Verification items for the finished model (mm, model axes). Face numbers are marked on the shaded views. Give positions to 0.01 mm unless a question says otherwise; leave off trailing zeros. Loops run counter-clockwise (first coordinate to the right, second up) from the corner with the lowest first, then second, coordinate; pieces in that order, holes last. Notation, with made-up numbers: (69, -40) - (103, -40) arc R22 cw to (103, -3) - close; hole circle Ø6 at (49.25, -5). An arc over 180 degrees is marked (long way). Put each result on its own line as item: value. Start each with the question number.
```python
from build123d import *

# Parameters (mm, degrees)
F0_W     = 50
F0_H     = 24
F0_R     = 2.75
F1_DEPTH = 4
F2_SIZE  = 7.62


with BuildPart() as f1:
    # F0 (on Top) → F1 (new body)
    with BuildSketch(Plane.XY):
        Rectangle(F0_W, F0_H)
        with Locations((-12.5, 0)):
            Circle(F0_R, mode=Mode.SUBTRACT)
        with BuildLine():
            ThreePointArc((15.2468, 0), (12.4968, -2.75), (9.7468, 0))
            ThreePointArc((9.7468, 0), (12.4968, 2.75), (15.2468, 0))
        make_face(mode=Mode.SUBTRACT)
    extrude(amount=F1_DEPTH)

    # F2
    f2_edges = [f1.edges().sort_by_distance(p)[0] for p in [
        (-25, 12, 2),
        (-25, -12, 2),
        (25, -12, 2),
        (25, 12, 2),
    ]]
    chamfer(f2_edges, length=F2_SIZE)


solid = f1.part
```
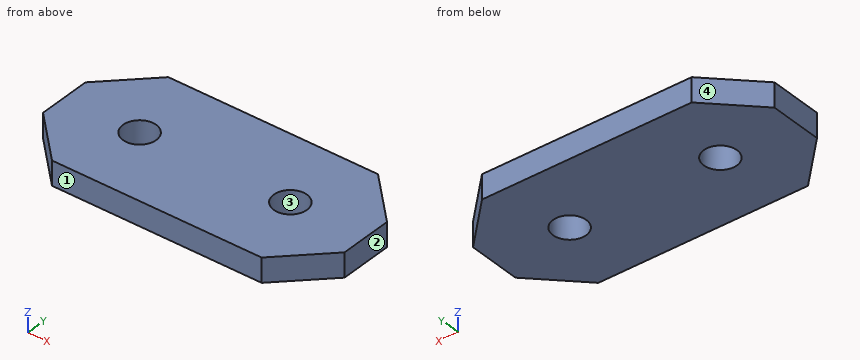
1) Section check B-B, the plane z = 2.7. Enter the section's corners in (x, y).
2) Depth check by flat-ended pin: P1, Ø7, axis at x = 12.5, y = 0, coming from the -Z side; P2, Ø4.5, axis at x = -12.5, y = 0, coming from the +Z side. Enter the tip coordinate at first touch or a pass-through.
3) Draft check along X on the marked faces 1, 2, 3 and 4. Enter one of: pulls with the +X half, pulls with the -X half, needs draft (parallel to the pull), parting line crosses it, or undercut.
4) Section check C-C, the plane x = -12.5. Enter the section's corners in (y, z).
5) Section check D-D, the plane y = 8.75. Enter the section's corners in (x, z).
6) Scan lines: line 1 along Y through (x, z) = (-12.5, 1.35); line 2 along X through (y, z) = (-0.75, 2.55); line 3 along Y through (x, z) = (-15, 1.8). Record each from-to range of solid material in increasing order. Write a range as from..to.
7) Section check A-A, the plane y = 0. Enter the section's corners in (x, z), plus the area to 3 significant figures.
Results are:
1. outline: (-25, -4.38) - (-17.38, -12) - (17.38, -12) - (25, -4.38) - (25, 4.38) - (17.38, 12) - (-17.38, 12) - (-25, 4.38) - close; hole circle Ø5.5 at (-12.5, 0); hole circle Ø5.5 at (12.5, 0)
2. P1: stops at z = 0
2. P2: passes through
3. face 1: needs draft
3. face 2: pulls with the +X half
3. face 3: undercut
3. face 4: pulls with the -X half
4. outline: (-12, 0) - (-2.75, 0) - (-2.75, 4) - (-12, 4) - close; (2.75, 0) - (12, 0) - (12, 4) - (2.75, 4) - close
5. outline: (-20.63, 0) - (20.63, 0) - (20.63, 4) - (-20.63, 4) - close
6. line 1: y = -12..-2.75, 2.75..12
6. line 2: x = -25..-15.15, -9.85..9.85, 15.14..25
6. line 3: y = -12..-1.15, 1.15..12
7. outline: (-25, 0) - (-15.25, 0) - (-15.25, 4) - (-25, 4) - close; (-9.75, 0) - (9.75, 0) - (9.75, 4) - (-9.75, 4) - close; (15.25, 0) - (25, 0) - (25, 4) - (15.25, 4) - close
7. area: 156 mm2
